Input: part model. Units: mm. Frame: model coordinates. A direction names the side the tool comes from. Round coordinates to 2 decimals unless told otherwise and drop trailing zeros. Order: outer loops, then holes, each group sorted by start corner. A loop starts at its lowest first (then second) coordinate and runs counter-clockwise, first axis right, second up.
Item 1: Cut plane A-A on y = -57. Output: boundary loops of the cut face in (x, z).
Item 2: First-contact query: pin 1 (0.5 mm diameter, centred on x = 1, z = -2, fed in from +Y); pin 2 (1.5 mm diameter, centred on x = 0, y = -89, fed in from -Z). Flat tips, straight axial feed; report the tip coordinate or a pass-through.
Item 3: Line query: L1, parallel to Z at x = 2.15, y = -2.5; L2, parallel to X at y = -50, z = 1.3. Output: solid intervals per line, ascending.
Item 4: Reachability of faces 1 (the flat face through (0, -63, 1.5)), 2 (the flat face through (1, -58, -2.5)) from +Z, -Z, +X, -X, +Y, -Y: full face, straight path, thin tool, end or side. Return the list, or none.
Item 5: Mould query, pull axis X, two halves, no side actions, for faces 3 (the flat face through (1.5, -60, 0)), 4 (the flat face through (2.5, -58, 0)), 5 (the flat face through (0, -118, 2)). Classes: released by +X, released by -X, zero draft, split by the parting line, or undercut.
```python
from build123d import *

# Parameters (mm, degrees)
F0_W     = 5
F0_H     = 5
F1_DEPTH = 118
F2_W     = 1
F2_H     = 1
F3_DEPTH = 118.001
F4_R     = 0.5
F5_DEPTH = 5.001
F6_R     = 0.5
F7_DEPTH = 5.001
F8_W     = 3
F8_H     = 6
F9_DEPTH = 5.001


with BuildPart() as f1:
    # F0 (on Front) → F1 (new body)
    with BuildSketch(Plane.XZ):
        Rectangle(F0_W, F0_H)
    extrude(amount=F1_DEPTH)

    # F2 (on face) → F3 (cut, through all)
    with BuildSketch(Plane.XZ.offset(118)):
        Polygon((0.5, -1.5), (1.5, -1.5), (1.5, 1.5), (-1.5, 1.5), (-1.5, -1.5), (-0.5, -1.5), align=None)
        with Locations((0, -2)):
            Rectangle(F2_W, F2_H)
    extrude(amount=-F3_DEPTH, mode=Mode.SUBTRACT)

    # F4 (on face) → F5 (cut, through all)
    with BuildSketch(Plane.YZ.offset(2.5)):
        with Locations((-79.5, 0)):
            Circle(F4_R)
    extrude(amount=-F5_DEPTH, mode=Mode.SUBTRACT)

    # F6 (on face) → F7 (cut, through all)
    with BuildSketch(Plane.YZ.offset(2.5)):
        with Locations((-2.5, 0)):
            Circle(F6_R)
    extrude(amount=-F7_DEPTH, mode=Mode.SUBTRACT)

    # F8 (on face) → F9 (cut, through all)
    with BuildSketch(Plane.XY.offset(2.5)):
        with Locations((0, -3)):
            Rectangle(F8_W, F8_H)
    extrude(amount=-F9_DEPTH, mode=Mode.SUBTRACT)


solid = f1.part
```
From the geometry:
1. outline: (-2.5, -2.5) - (-0.5, -2.5) - (-0.5, -1.5) - (-1.5, -1.5) - (-1.5, 1.5) - (1.5, 1.5) - (1.5, -1.5) - (0.5, -1.5) - (0.5, -2.5) - (2.5, -2.5) - (2.5, 2.5) - (-2.5, 2.5) - close
2. pin 1: stops at y = -6
2. pin 2: stops at z = -2.5
3. L1: z = -2.5 to -0.5, 0.5 to 2.5
3. L2: x = -2.5 to -1.5, 1.5 to 2.5
4. face 1: +Y, -Y
4. face 2: -Z, +X, -X, +Y, -Y
5. face 3: undercut
5. face 4: released by +X
5. face 5: zero draft
